from build123d import *

# Parameters (mm, degrees)
SKETCH1_R           = 30
BOSS_EXTRUDE1_DEPTH = 5
SKETCH2_R           = 32.5
BOSS_EXTRUDE2_DEPTH = 1
SKETCH3_R           = 21.5
CUT_EXTRUDE1_DEPTH  = 25
SKETCH4_R           = 1.6
CUT_EXTRUDE2_DEPTH  = 25


with BuildPart() as part:
    # Sketch1 → Boss-Extrude1 (new body)
    with BuildSketch(Plane(origin=(0, 0, 0), x_dir=(1, 0, 0), z_dir=(0, 1, 0))):
        with Locations(Location((0, 0, 0), (0, 0, 270))):
            Circle(SKETCH1_R)
    extrude(amount=BOSS_EXTRUDE1_DEPTH)

    # Sketch2 → Boss-Extrude2 (add)
    with BuildSketch(Plane(origin=(0, 5, 0), x_dir=(1, 0, 0), z_dir=(0, 1, 0))):
        with Locations(Location((0, 0, 0), (0, 0, 270))):
            Circle(SKETCH2_R)
    extrude(amount=-BOSS_EXTRUDE2_DEPTH)

    # Sketch3 → Cut-Extrude1 (cut)
    with BuildSketch(Plane.XZ):
        with Locations(Location((0, 0, 0), (0, 0, 270))):
            Circle(SKETCH3_R)
    extrude(amount=-CUT_EXTRUDE1_DEPTH, mode=Mode.SUBTRACT)

    # Sketch4 → Cut-Extrude2 (cut)
    with BuildSketch(Plane(origin=(0, 5, 0), x_dir=(1, 0, 0), z_dir=(0, 1, 0))):
        with Locations(Location((0, 25, 0), (0, 0, 270))):
            Circle(SKETCH4_R)
        with Locations(Location((21.650635095, 12.5, 0), (0, 0, 270))):
            Circle(SKETCH4_R)
        with Locations(Location((21.650635095, -12.5, 0), (0, 0, 270))):
            Circle(SKETCH4_R)
        with Locations(Location((0, -25, 0), (0, 0, 270))):
            Circle(SKETCH4_R)
        with Locations(Location((-21.650635095, -12.5, 0), (0, 0, 270))):
            Circle(SKETCH4_R)
        with Locations(Location((-21.650635095, 12.5, 0), (0, 0, 270))):
            Circle(SKETCH4_R)
    extrude(amount=-CUT_EXTRUDE2_DEPTH, mode=Mode.SUBTRACT)


solid = part.part
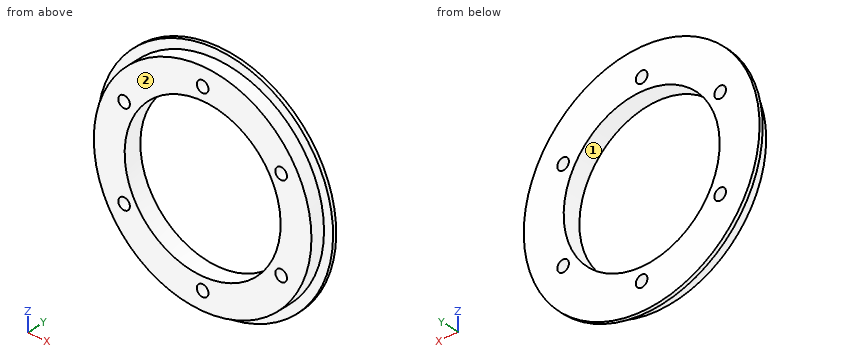
CAD build for the part. Positions are in the model's coordinates, mm. Face numbers are marked on the shaded views. Give positions to 0.01 mm unless a question says otherwise; leave off trailing zeros. Order: outer loops, then holes, each group sorted by start corner. A loop starts at its lowest first (then second) coordinate and runs counter-clockwise, first axis right, second up. Notation, with made-up numbers: (-2.75, 30) - (21.25, 30) arc R16 cw to (21.25, 44) - close; hole circle Ø5 at (34, -1.75). An arc over 180 degrees is marked (long way). Answer in a Markdown table with one row per item.
1. Flat gauge pins, fed straight in: pin 1 (10 mm diameter, centred on x = -8.5, z = 18, fed in from +Y); pin 2 (2 mm diameter, centred on y = 2, z = 10.5, fed in from +X). Where does each tip first touch, or does it go through?
Data:
| item | result |
|---|---|
| pin 1 | stops at y = 5 |
| pin 2 | stops at x = 28.46 |
2. Saw through at D-D, the plane y = 2.2. Give the cut face in (x, z), plus the area to 3 significant figures.
Data:
| item | result |
|---|---|
| outline | circle Ø60 at (0, 0); hole circle Ø3.2 at (-21.65, -12.5); hole circle Ø3.2 at (-21.65, 12.5); hole circle Ø43 at (0, 0); hole circle Ø3.2 at (0, -25); hole circle Ø3.2 at (0, 25); hole circle Ø3.2 at (21.65, -12.5); hole circle Ø3.2 at (21.65, 12.5) |
| area | 1,330 mm² |
3. Saw through at A-A, the plane z = 0. Give the cut face in (x, y).
Data:
| item | result |
|---|---|
| outline | (-32.5, 4) - (-30, 4) - (-30, 0) - (-21.5, 0) - (-21.5, 5) - (-32.5, 5) - close; (21.5, 0) - (30, 0) - (30, 4) - (32.5, 4) - (32.5, 5) - (21.5, 5) - close |
4. Pull direction Z, two halves, no side cores. Call the marked faces 1 and 2: pulls with the +Z half, pulls with the -Z half, needs draft (parallel to the pull), parting line crosses it, or undercut.
Data:
| item | result |
|---|---|
| face 1 | undercut |
| face 2 | needs draft |
5. Probe probe 1 along X at (y, z) = (1.75, 12.5); probe 2 along Z at (x, y) = (1, 3); probe 3 along Z at (x, y) = (0.5, 4.75). List the from-to ranges inside material, lowest first. Write a range as [from, to].
Data:
| item | result |
|---|---|
| probe 1 | x = [-27.27, -23.25], [-20.05, -17.49], [17.49, 20.05], [23.25, 27.27] |
| probe 2 | z = [-29.98, -26.25], [-23.75, -21.48], [21.48, 23.75], [26.25, 29.98] |
| probe 3 | z = [-32.5, -26.52], [-23.48, -21.49], [21.49, 23.48], [26.52, 32.5] |
6. Saw through at C-C, the plane x = 12.5. Give the cut face in (y, z).
Data:
| item | result |
|---|---|
| outline | (0, -27.27) - (4, -27.27) - (4, -30) - (5, -30) - (5, -17.49) - (0, -17.49) - close; (0, 17.49) - (5, 17.49) - (5, 30) - (4, 30) - (4, 27.27) - (0, 27.27) - close |
7. Saw through at B-B, the plane x = 0. Give the cut face in (y, z).
Data:
| item | result |
|---|---|
| outline | (0, -30) - (4, -30) - (4, -32.5) - (5, -32.5) - (5, -26.6) - (0, -26.6) - close; (0, -23.4) - (5, -23.4) - (5, -21.5) - (0, -21.5) - close; (0, 21.5) - (5, 21.5) - (5, 23.4) - (0, 23.4) - close; (0, 26.6) - (5, 26.6) - (5, 32.5) - (4, 32.5) - (4, 30) - (0, 30) - close |
